from build123d import *

# Parameters (mm, degrees)
ESQUISSE1_W             = 8
ESQUISSE1_H             = 3
ESQUISSE1_W_2           = 3
ESQUISSE1_H_2           = 8
BOSS_EXTRU_1_DEPTH      = 6
CONG_1_R                = 10
ESQUISSE2_W             = 8
ESQUISSE2_H             = 6
ENL_V_MAT_EXTRU_1_DEPTH = 3


with BuildPart() as part:
    # Esquisse1 → Boss.-Extru.1 (new body)
    with BuildSketch(Plane.XY):
        Polygon((-60, 35), (-69, 35), (-77, 35), (-80, 35), (-65, 15), (-15, 15), (-15, 0), (0, 0), (0, 8), (0, 13), (0, 21), (0, 26), (0, 34), (0, 35), (-1, 35), (-9, 35), (-18, 35), (-26, 35), (-35, 35), (-43, 35), (-52, 35), align=None)
        with Locations((-56, 36.5)):
            Rectangle(ESQUISSE1_W, ESQUISSE1_H)
        with Locations((-39, 36.5)):
            Rectangle(ESQUISSE1_W, ESQUISSE1_H)
        with Locations((-22, 36.5)):
            Rectangle(ESQUISSE1_W, ESQUISSE1_H)
        with Locations((-5, 36.5)):
            Rectangle(ESQUISSE1_W, ESQUISSE1_H)
        with Locations((1.5, 30)):
            Rectangle(ESQUISSE1_W_2, ESQUISSE1_H_2)
        with Locations((1.5, 17)):
            Rectangle(ESQUISSE1_W_2, ESQUISSE1_H_2)
        with Locations((1.5, 4)):
            Rectangle(ESQUISSE1_W_2, ESQUISSE1_H_2)
        with Locations((-73, 36.5)):
            Rectangle(ESQUISSE1_W, ESQUISSE1_H)
    extrude(amount=BOSS_EXTRU_1_DEPTH)

    # Congé1
    # the kernel refuses this fillet: 10 mm, written as the material it takes off along each edge
    with BuildSketch(Plane(origin=(-80, 35, -20.748076809), x_dir=(1, 0, 0), z_dir=(0, 0, 1))) as cong_1_piece_1:
        with BuildLine():
            CenterArc((12.979538434, -0.639384579), CONG_1_R, 176.334095535, 40.535802111)
            Line((4.979538434, -6.639384579), (4.819538434, -6.759384579))
            Line((4.819538434, -6.759384579), (-0.16, -0.12))
            Line((-0.16, -0.12), (0, 0.2))
            ThreePointArc((0, 0.2), (1.5, 0.2), (2.800409231, 0.012787692))
            Line((2.800409231, 0.012787692), (3, 0))
        make_face()
    extrude(amount=47.496153619, mode=Mode.SUBTRACT)

    # Esquisse2 → Enlèv. mat.-Extru.1 (cut)
    with BuildSketch(Plane(origin=(0, 38, 0), x_dir=(1, 0, 0), z_dir=(0, 1, 0))):
        with Locations((-39, -3)):
            Rectangle(ESQUISSE2_W, ESQUISSE2_H)
    extrude(amount=-ENL_V_MAT_EXTRU_1_DEPTH, mode=Mode.SUBTRACT)


solid = part.part
Design review of the part built by this model. Coordinates are the model's own, in mm. A direction names the side the tool comes from. Coordinates: 2 decimals unless noted, no trailing zeros. Order: outer loops, then holes, each group sorted by start corner. A loop starts at its lowest first (then second) coordinate and runs counter-clockwise, first axis right, second up.
Item 1: For faces 1 (the flat face through (-1, 36, 3)), 2 (the flat face through (0, 23, 3)), 3 (the flat face through (-26, 36, 3)), list the 3-axis set-ups (+Z, -Z, +X, -X, +Y, -Y) from which the entire face can be reached by the end or side of a thin tool; tool diameter is ignored.
Item 2: Take a section at C-C, the plane y = 20. Write out the cut boundary in (x, z).
Item 3: For pin 1 Ø1.5 at (y, z) = (36.5, 4) entering from +X; pin 2 Ø3 at (x, z) = (-65.5, 2) entering from +Y; pin 3 Ø3 at (y, z) = (7.5, 3) entering from -X, all flat-tipped, find the tip position at first contact; note any pin that passes through.
Item 4: Take a section at B-B, the plane x = -22.5. Write out the cut boundary in (y, z).
Item 5: The part is to be moulded in two halves that separate along X. For faces 4 (the flat face through (-13, 35, 3)), 5 (the flat face through (-60, 36, 3)), 6 (the flat face through (-73, 38, 3)), 7 (the flat face through (0, 10, 3)), say which applies: pulls with the +X half, pulls with the -X half, needs draft (parallel to the pull), parting line crosses it, or undercut.
Item 6: For line 1 (X direction, y = 12.5, z = 5.55); line 2 (X direction, y = 5.5, z = 5.45); line 3 (Y direction, x = -46, z = 5.45), list the stretches that pass through material, from the lowest coordinate up.
The answers:
1. face 1: +Z, -Z, +X, +Y
1. face 2: +Z, -Z, +X
1. face 3: +Z, -Z, +Y
2. outline: (-68.75, 0) - (3, 0) - (3, 6) - (-68.75, 6) - close
3. pin 1: stops at x = -1
3. pin 2: stops at y = 35
3. pin 3: stops at x = -15
4. outline: (15, 0) - (38, 0) - (38, 6) - (15, 6) - close
5. face 4: undercut
5. face 5: undercut
5. face 6: needs draft
5. face 7: pulls with the +X half
6. line 1: x = -15 to 0
6. line 2: x = -15 to 3
6. line 3: y = 15 to 35
